Design review of the part built by this model. Coordinates are the model's own, in mm. Give positions to 0.01 mm unless a question says otherwise; leave off trailing zeros. Loops run counter-clockwise (first coordinate to the right, second up) from the corner with the lowest first, then second, coordinate; pieces in that order, holes last.
from build123d import *

# Parameters (mm, degrees)
SKETCH_1_R               = 60
SKETCH_1_R_2             = 45
EXTRUDE_1_DEPTH          = 2
SKETCH_2_R               = 1.5
CUT_EXTRUDE_1_DEPTH      = 50
PATTERN_CIRCULAR_1_COUNT = 8


with BuildPart() as part:
    # 草图1 → 凸台-拉伸1 (new body)
    with BuildSketch(Plane(origin=(0, 0, 0), x_dir=(1, 0, 0), z_dir=(0, 1, 0))):
        with Locations(Location((0, 0, 0), (0, 0, 270))):
            Circle(SKETCH_1_R)
        with Locations(Location((0, 0, 0), (0, 0, 270))):
            Circle(SKETCH_1_R_2, mode=Mode.SUBTRACT)
    extrude(amount=EXTRUDE_1_DEPTH)

    # 草图2 → 切除-拉伸1 (cut)
    with BuildSketch(Plane.XZ):
        with Locations(Location((-51.989320621, 1.053822248, 0), (0, 0, 270))):
            Circle(SKETCH_2_R)
    cut_extrude_1 = extrude(amount=-CUT_EXTRUDE_1_DEPTH, mode=Mode.SUBTRACT)

    # 阵列(圆周)1: 切除-拉伸1 ×8 about axis
    pattern_circular_1_axis = Axis((0, 0, 0), (0, 1, 0))
    for i in range(1, PATTERN_CIRCULAR_1_COUNT):
        add(cut_extrude_1.rotate(pattern_circular_1_axis, i * 360 / PATTERN_CIRCULAR_1_COUNT), mode=Mode.SUBTRACT)


solid = part.part
Q1. Insertion check: pin 1 (1 mm diameter, centred on y = 1, z = 37, fed in from -X). The pin has a flat end and moves straight along its axis. Give the tip position at first contact, or say it passes through.
Results:
pin 1: stops at x = -47.62
Q2. Take a section at C-C (y = 1.45). Give the number of separate pieces and of enclosed holes in the cut face, plus the area to 3 significant figures.
Results:
separate pieces: 1
enclosed holes: 9
area: 4,890 mm2
Q3. Draft analysis for pull direction Z (two halves, no side actions). For faces 1 (the face through (45, 0, 9)), 2 (the face through (2.64, 0.99, -59.94)), 3 (the face through (-35.693, 0.986, 36.043)), state which applies: pulls with the +Z half, pulls with the -Z half, needs draft (parallel to the pull), parting line crosses it, or undercut.
Results:
face 1: needs draft
face 2: parting line crosses it
face 3: undercut
Q4. Wall thickness on line 1 (X direction, y = 0.65, z = 0); line 2 (X direction, y = 0.9, z = -36.5); line 3 (Z direction, x = -6, y = 1.25): over which ranges is each line inside the solid? List them lowest first.
Results:
line 1: x = -60 to -53.06, -50.92 to -45, 45 to 50.92, 53.06 to 60
line 2: x = -47.62 to -38.93, -36.09 to -26.32, 26.32 to 34.91, 37.13 to 47.62
line 3: z = -59.7 to -44.6, 44.6 to 59.7
Q5. Take a section at A-A (x = -27). Give the boundary of the cut face in (y, z).
Results:
outline: (0, -53.58) - (2, -53.58) - (2, -36) - (0, -36) - close; (0, 36) - (2, 36) - (2, 53.58) - (0, 53.58) - close
Q6. Take a section at B-B (z = -33). Give the boundary of the cut face in (x, y), plus the area to 3 significant figures.
Results:
outline: (-50.11, 0) - (-30.59, 0) - (-30.59, 2) - (-50.11, 2) - close; (30.59, 0) - (50.11, 0) - (50.11, 2) - (30.59, 2) - close
area: 78.1 mm2
